Source: CAD feature listing. Evaluate the final solid. Frame: model axes, mm. A direction names the side the tool comes from. Give positions to 0.01 mm unless a question says otherwise; leave off trailing zeros. Write each loop counter-clockwise with the first axis right and the second up, starting at its lowest first coordinate (ties: lowest second). Pieces come first, ordered by that corner, then holes. Notation, with made-up numbers: (66.25, 26.25) -> (76.25, 26.25) arc R25 cw to (76.25, 58.25) -> close; hole circle Ø11 at (72, 70). An arc over 180 degrees is marked (long way). Write item = value, one per line.
from build123d import *

# Parameters (mm, degrees)
SKETCH_1_W          = 68
SKETCH_1_H          = 40
EXTRUDE_1_DEPTH     = 20
SKETCH_2_W          = 38
SKETCH_2_H          = 18
CUT_EXTRUDE_1_DEPTH = 74.647810558
SKETCH_3_R          = 2
CUT_EXTRUDE_2_DEPTH = 1
SKETCH_4_R          = 14.8
SKETCH_4_R_2        = 1.5
CUT_EXTRUDE_3_DEPTH = 1
MM_PRESS_1_D        = 4
MM_PRESS_1_DEPTH    = 1
MM_PRESS_1_TIP      = 1.201721238


with BuildPart() as part:
    # 草图1 → 凸台-拉伸1 (new body)
    with BuildSketch(Plane(origin=(0, 0, 0), x_dir=(1, 0, 0), z_dir=(0, 1, 0))):
        Rectangle(SKETCH_1_W, SKETCH_1_H)
    extrude(amount=EXTRUDE_1_DEPTH)

    # 草图2 → 切除-拉伸1 (cut, through all)
    with BuildSketch(Plane(origin=(34, 0, 0), x_dir=(0, 0, -1), z_dir=(1, 0, 0))):
        with Locations((0, 10)):
            Rectangle(SKETCH_2_W, SKETCH_2_H)
    extrude(amount=-CUT_EXTRUDE_1_DEPTH, mode=Mode.SUBTRACT)

    # 草图3 → 切除-拉伸2 (cut)
    with BuildSketch(Plane.XZ):
        with Locations(Location((-21, 0, 0), (0, 0, 270))):
            Circle(SKETCH_3_R)
        with Locations(Location((21, 0, 0), (0, 0, 270))):
            Circle(SKETCH_3_R)
    extrude(amount=-CUT_EXTRUDE_2_DEPTH, mode=Mode.SUBTRACT)

    # 草图4 → 切除-拉伸3 (cut)
    with BuildSketch(Plane(origin=(0, 20, 0), x_dir=(1, 0, 0), z_dir=(0, 1, 0))):
        with Locations(Location((0, 0, 0), (0, 0, 270))):
            Circle(SKETCH_4_R)
        with Locations(Location((-17, 0, 0), (0, 0, 270))):
            Circle(SKETCH_4_R_2)
        with Locations(Location((17, 0, 0), (0, 0, 270))):
            Circle(SKETCH_4_R_2)
    extrude(amount=-CUT_EXTRUDE_3_DEPTH, mode=Mode.SUBTRACT)

    # 大小mm Press 暗销孔1
    with Locations(Plane(origin=(16.970562748, 20, 16.970562748), x_dir=(0, 0, 1), z_dir=(0, 1, 0))):
        with Locations((0, 0), (0, -33.941125496), (-33.941125496, -33.941125496), (-33.941125496, 0)):
            Hole(MM_PRESS_1_D / 2, depth=MM_PRESS_1_DEPTH)
            with Locations((0, 0, -(MM_PRESS_1_DEPTH + MM_PRESS_1_TIP / 2))):  # 118° drill point
                Cone(0, MM_PRESS_1_D / 2, MM_PRESS_1_TIP, mode=Mode.SUBTRACT)


solid = part.part
(1) Pull-direction query (X, two-part tool) for faces 5 (the face through (0, 10, 20)), 6 (the face through (-16.88, 19.49, 18.97)), 7 (the face through (-34, 19.6, 1.6)); classes: pulls with the +X half, pulls with the -X half, needs draft (parallel to the pull), parting line crosses it, or undercut.
Values follow:
face_5 = needs draft
face_6 = undercut
face_7 = pulls with the -X half
(2) First-contact query: pin 1 (18 mm diameter, centred on x = 0, z = 0, fed in from +Y). Flat tip, straight axial feed; report the tip coordinate or a pass-through.
Values follow:
pin_1 = 1
(3) Material intervals for line 1 (Y direction, x = -23, z = -14.5); line 2 (Z direction, x = 1.5, y = 4); line 3 (X direction, y = 0.6, z = 0), sorted ascending.
Values follow:
line_1 = 0 to 1, 19 to 20
line_2 = -20 to -19, 19 to 20
line_3 = -34 to -23, -19 to 19, 23 to 34
(4) Section query D-D (x = -21). Return loops of the section in (y, z), plus the area to 3 significant figures.
Values follow:
outline = (0, -20) -> (20, -20) -> (20, 20) -> (0, 20) -> (0, 2) -> (1, 2) -> (1, 19) -> (19, 19) -> (19, -19) -> (1, -19) -> (1, -2) -> (0, -2) -> close
area = 112 mm2
(5) Section query A-A (y = 12). Return loops of the section in (x, z), plus the area to 3 significant figures.
Values follow:
outline = (-34, -20) -> (34, -20) -> (34, -19) -> (-34, -19) -> close; (-34, 19) -> (34, 19) -> (34, 20) -> (-34, 20) -> close
area = 136 mm2
(6) Access query for faces 1 (the face through (-19.017, 0.493, 0.26)), 2 (the face through (8, 19, 13)), 3 (the face through (17.06, 19.49, 18.97)), 4 (the face through (34, 19.6, 1.6)). Directions: +Z, -Z, +X, -X, +Y, -Y. A direction counts if a zero-diameter tool reaches every point of the face in a straight line with its end or side. Return the directions, or none.
Values follow:
face_1 = -Y
face_2 = +X, -X
face_3 = +Y
face_4 = +Z, -Z, +X, +Y, -Y
(7) Section query C-C (z = -16). Return loops of the section in (x, y).
Values follow:
outline = (-34, 0) -> (34, 0) -> (34, 1) -> (-34, 1) -> close; (-34, 19) -> (-18.72, 19) -> (-18.72, 20) -> (-34, 20) -> close; (-15.22, 19) -> (15.22, 19) -> (15.22, 20) -> (-15.22, 20) -> close; (18.72, 19) -> (34, 19) -> (34, 20) -> (18.72, 20) -> close
(8) Section query B-B (z = 0). Return loops of the section in (x, y).
Values follow:
outline = (-34, 0) -> (-23, 0) -> (-23, 1) -> (-34, 1) -> close; (-34, 19) -> (-18.5, 19) -> (-18.5, 20) -> (-34, 20) -> close; (-19, 0) -> (19, 0) -> (19, 1) -> (-19, 1) -> close; (-15.5, 19) -> (-14.8, 19) -> (-14.8, 20) -> (-15.5, 20) -> close; (14.8, 19) -> (15.5, 19) -> (15.5, 20) -> (14.8, 20) -> close; (18.5, 19) -> (34, 19) -> (34, 20) -> (18.5, 20) -> close; (23, 0) -> (34, 0) -> (34, 1) -> (23, 1) -> close
